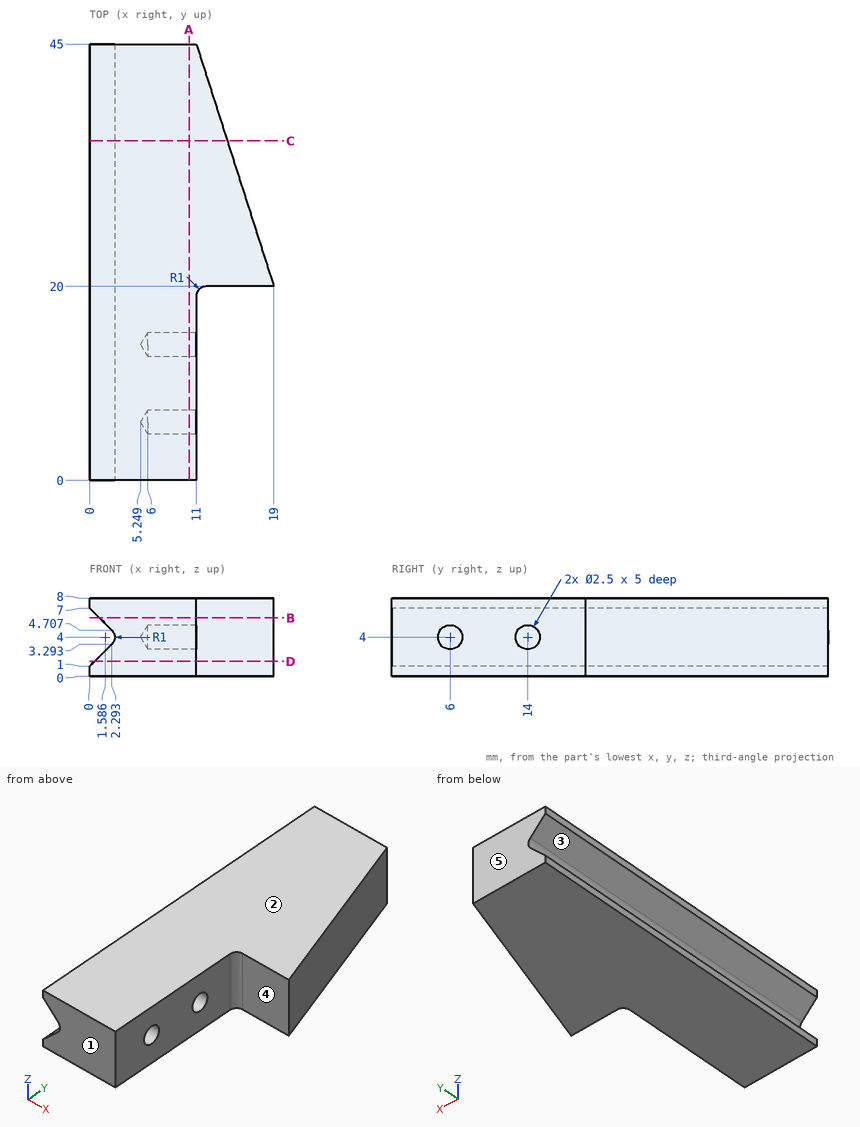
Source: three-view drawing plus pictorial views. Frame: mm from the lowest corner of the part. A direction names the side the tool comes from. Round coordinates to 2 decimals unless told otherwise and drop trailing zeros. Order: outer loops, then holes, each group sorted by start corner. A loop starts at its lowest first (then second) coordinate and runs counter-clockwise, first axis right, second up. Notation, with made-up numbers: (-8.75, 28) - (27.25, 28) arc R17 ccw to (27.25, 40) - close; hole circle Ø4 at (-26.5, -4.5). An arc over 180 degrees is marked (long way). Use a Markdown table: item, result.
1. Access query for the marked faces 4 and 5. Directions: +Z, -Z, +X, -X, +Y, -Y. A direction counts if a zero-diameter tool reaches every point of the face in a straight line with its end or side. Return the directions, or none.
Evaluation:
| item | result |
|---|---|
| face 4 | +Z, -Z, +X, -Y |
| face 5 | +Z, -Z, +X, -X, +Y |
2. Section A-A on x = 10.25. Return the cut outline in (y, z).
Evaluation:
| item | result |
|---|---|
| outline | (0, 0) - (45, 0) - (45, 8) - (0, 8) - close; hole circle Ø2.5 at (6, 4); hole circle Ø2.5 at (14, 4) |
3. Section D-D on z = 1.5. Return the cut outline in (x, y).
Evaluation:
| item | result |
|---|---|
| outline | (0.5, 0) - (11, 0) - (11, 19) arc R1 cw to (12, 20) - (19, 20) - (11, 45) - (0.5, 45) - close |
4. Section B-B on z = 6. Return the cut outline in (x, y), then the cut area to 3 significant figures.
Evaluation:
| item | result |
|---|---|
| outline | (1, 0) - (11, 0) - (11, 19) arc R1 cw to (12, 20) - (19, 20) - (11, 45) - (1, 45) - close |
| area | 550 mm^2 |
5. Mould query, pull axis Z, two halves, no side actions, for the marked faces 1, 2 and 3. Classes: +Z half, -Z half, draft (parallel to the pull), parting line (faces both ways), or undercut.
Evaluation:
| item | result |
|---|---|
| face 1 | draft |
| face 2 | +Z half |
| face 3 | undercut |
6. Material intervals for probe 1 along Y at (x, z) = (8, 4); probe 2 along Z at (x, y) = (2, 25); probe 3 along X at (y, z) = (12.5, 6), sorted ascending.
Evaluation:
| item | result |
|---|---|
| probe 1 | 0 to 4.75, 7.25 to 12.75, 15.25 to 45 |
| probe 2 | 0 to 3, 5 to 8 |
| probe 3 | 1 to 11 |
7. First-contact query: pin 1 (3 mm diameter, centred on y = 20.5, z = 5.5, fed in from +X); pin 2 (4 mm diameter, centred on y = 10.5, z = 5.5, fed in from +X); pin 3 (1.5 mm diameter, centred on y = 6, z = 4, fed in from -X); pin 4 (2 mm diameter, centred on x = 16, z = 2.5, fed in from -Y). Flat tips, straight axial feed; report the tip coordinate or a pass-through.
Evaluation:
| item | result |
|---|---|
| pin 1 | x = 19 |
| pin 2 | x = 11 |
| pin 3 | x = 2.25 |
| pin 4 | y = 20 |
8. Section C-C on y = 35. Return the cut outline in (x, z).
Evaluation:
| item | result |
|---|---|
| outline | (0, 0) - (14.2, 0) - (14.2, 8) - (0, 8) - (0, 7) - (2.29, 4.71) arc R1 cw to (2.29, 3.29) - (0, 1) - close |
